Verification items for the finished model (mm, model axes). Coordinates: 2 decimals unless noted, no trailing zeros. Write each loop counter-clockwise with the first axis right and the second up, starting at its lowest first coordinate (ties: lowest second). Pieces come first, ordered by that corner, then holes. Notation, with made-up numbers: (49, 28.25) -> (66, 28.25) arc R22 cw to (66, 56.25) -> close; hole circle Ø10 at (0.5, 88.25). An arc over 180 degrees is marked (long way). Answer in a Markdown table with one row per item.
```python
from build123d import *

# Parameters (mm, degrees)
SKETCH1_R               = 120
BOSS_EXTRUDE1_DEPTH     = 600
CUT_EXTRUDE1_START      = -580
CUT_EXTRUDE1_DEPTH      = 580
CUT_EXTRUDE3_DEPTH      = 624.538290725
CUT_EXTRUDE3_DEPTH_BACK = 624.538290725


with BuildPart() as part:
    # Sketch1 → Boss-Extrude1 (new body)
    with BuildSketch(Plane(origin=(0, 0, 0), x_dir=(0, 0, -1), z_dir=(1, 0, 0))):
        Circle(SKETCH1_R)
    extrude(amount=BOSS_EXTRUDE1_DEPTH)

    # Sketch2 → Cut-Extrude1 (cut)
    with BuildSketch(Plane(origin=(600, 0, 0), x_dir=(0, 0, -1), z_dir=(1, 0, 0)).offset(CUT_EXTRUDE1_START)):
        with BuildLine():
            Line((-110, 0), (-120, 0))
            ThreePointArc((-120, 0), (0, 120), (120, 0))
            Line((120, 0), (110, 0))
            ThreePointArc((110, 0), (0, -110), (-110, 0))
        make_face()
    extrude(amount=CUT_EXTRUDE1_DEPTH, mode=Mode.SUBTRACT)

    # Sketch5 → Cut-Extrude3 (cut, two sides: drawn at the far end of the back side and taken through both)
    with BuildSketch(Plane.XY.offset(-CUT_EXTRUDE3_DEPTH_BACK)):
        with BuildLine():
            Line((303.579878798, 0), (600, 0))
            Line((600, 0), (600, -60))
            add(Edge.make_bspline(
                [(303.579878798, 0), (445.56940812, -63.340252394), (600, -60)],
                knots=[0, 0, 0, 1, 1, 1], degree=2))
        make_face()
    extrude(amount=CUT_EXTRUDE3_DEPTH + CUT_EXTRUDE3_DEPTH_BACK, mode=Mode.SUBTRACT)


solid = part.part
```
1. Section check B-B, the plane z = -13.5. Record the boundary of the cut face in (x, y), plus the area to 3 significant figures.
Geometry says:
| item | result |
|---|---|
| outline | (0, -119.24) -> (600, -119.24) -> (600, -109.17) -> (20, -109.17) -> (20, 119.24) -> (0, 119.24) -> close |
| area | 10,600 mm^2 |
2. Section check A-A, the plane y = -93. Record the boundary of the cut face in (x, z), plus the area to 3 significant figures.
Geometry says:
| item | result |
|---|---|
| outline | (0, -75.84) -> (600, -75.84) -> (600, -58.75) -> (20, -58.75) -> (20, 58.75) -> (600, 58.75) -> (600, 75.84) -> (0, 75.84) -> close |
| area | 22,900 mm^2 |
3. Thickness scan on line 1 (X direction, y = -50, z = 64); line 2 (Z direction, x = 493, y = -96); line 3 (Z direction, x = 231.5, y = -32). Record the ranges inside material, lowest first. Write a range as from..to.
Geometry says:
| item | result |
|---|---|
| line 1 | 0..20 |
| line 2 | -72..-53.7, 53.7..72 |
| line 3 | -115.65..-105.24, 105.24..115.65 |
4. Mould release check, pull along Z, two halves, no side actions. Record for faces 1 (the flat face through (600, -112, 0)), 2 (the cylindrical face through (305.94, -109.973, -2.419)), 3 (the cylindrical face through (295.8, -117.146, 26.014)): released by +Z, released by -Z, zero draft, split by the parting line, or undercut.
Geometry says:
| item | result |
|---|---|
| face 1 | zero draft |
| face 2 | undercut |
| face 3 | split by the parting line |
5. Section check D-D, the plane z = 74. Record the boundary of the cut face in (x, y).
Geometry says:
| item | result |
|---|---|
| outline | (0, -94.47) -> (600, -94.47) -> (600, -81.39) -> (20, -81.39) -> (20, 94.47) -> (0, 94.47) -> close |
6. Section check C-C, the plane x = 209. Record the boundary of the cut face in (y, z).
Geometry says:
| item | result |
|---|---|
| outline | (0, -120) -> (0, -110) arc R110 cw to (0, 110) -> (0, 120) arc R120 ccw to start |
7. Depth check by flat-ended pin: P1, Ø3, axis at y = 65, z = -17, coming from the +X side; P2, Ø4, axis at x = 364, y = -92, coming from the -Z side; P3, Ø8, axis at x = 498, z = 11.5, coming from the -Y side. Enter the tip coordinate at first touch or a pass-through.
Geometry says:
| item | result |
|---|---|
| P1 | x = 20 |
| P2 | z = -79.37 |
| P3 | y = -119.77 |
